Geometry: final body of the model. Coordinates: model frame, mm. Face numbers are marked on the shaded views. A direction names the side the tool comes from. Give positions to 0.01 mm unless a question says otherwise; leave off trailing zeros. Loops run counter-clockwise (first coordinate to the right, second up) from the corner with the lowest first, then second, coordinate; pieces in that order, holes last. Notation, with made-up numbers: (31, 0.5) -> (67, 0.5) arc R28 cw to (67, 18.5) -> close; hole circle Ø9 at (8, 85). An arc over 180 degrees is marked (long way). One line per item, written item: value. Start each with the question number.
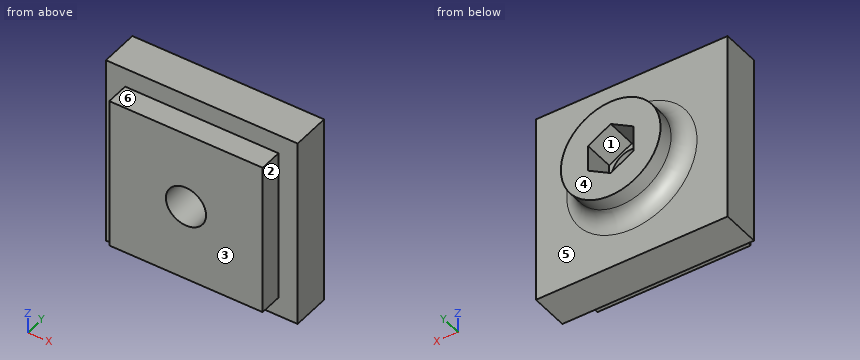
from build123d import *

# Parameters (mm, degrees)
SKETCH2_W               = 25
SKETCH2_H               = 25
BOSS_EXTRUDE1_DEPTH     = 5
SKETCH3_W               = 20
SKETCH3_H               = 20
BOSS_EXTRUDE2_DEPTH     = 3
SKETCH4_R               = 6.5
BOSS_EXTRUDE3_DEPTH     = 4
CUT_EXTRUDE1_DEPTH      = 22.365860619
CUT_EXTRUDE1_DEPTH_BACK = 22.365860619
SKETCH5_R               = 2.62
CUT_EXTRUDE2_DEPTH      = 4
FILLET1_R               = 2


with BuildPart() as part:
    # Sketch2 → Boss-Extrude1 (new body)
    with BuildSketch(Plane(origin=(0, 0, 0), x_dir=(1, 0, 0), z_dir=(0, 1, 0))):
        Rectangle(SKETCH2_W, SKETCH2_H)
    extrude(amount=BOSS_EXTRUDE1_DEPTH)

    # Sketch3 → Boss-Extrude2 (add)
    with BuildSketch(Plane.XZ):
        Rectangle(SKETCH3_W, SKETCH3_H)
    extrude(amount=BOSS_EXTRUDE2_DEPTH)

    # Sketch4 → Boss-Extrude3 (add)
    with BuildSketch(Plane(origin=(0, 5, 0), x_dir=(1, 0, 0), z_dir=(0, 1, 0))):
        with Locations(Location((0, 0, 0), (0, 0, 270))):
            Circle(SKETCH4_R)
    extrude(amount=BOSS_EXTRUDE3_DEPTH)

    # Sketch5 → Cut-Extrude1 (cut, two sides: drawn at the far end of the back side and taken through both)
    with BuildSketch(Plane(origin=(0, 9, 0), x_dir=(1, 0, 0), z_dir=(0, 1, 0)).offset(-CUT_EXTRUDE1_DEPTH_BACK)):
        with Locations(Location((0, 0, 0), (0, 0, 270))):
            Circle(SKETCH5_R)
    extrude(amount=CUT_EXTRUDE1_DEPTH + CUT_EXTRUDE1_DEPTH_BACK, mode=Mode.SUBTRACT)

    # Sketch6 → Cut-Extrude2 (cut)
    with BuildSketch(Plane(origin=(0, 9, 0), x_dir=(1, 0, 0), z_dir=(0, 1, 0))):
        Polygon((0, 3.406366588), (-2.95, 1.703183294), (-2.95, -1.703183294), (0, -3.406366588), (2.95, -1.703183294), (2.95, 1.703183294), align=None)
    extrude(amount=-CUT_EXTRUDE2_DEPTH, mode=Mode.SUBTRACT)

    # Fillet1
    fillet1_edges = [part.edges().sort_by_distance(p)[0] for p in [
        (0, 5, -6.5),
    ]]
    fillet(fillet1_edges, radius=FILLET1_R)


solid = part.part
Item 1: Section D-D, the plane z = -9.25. Output: boundary loops of the cut face in (x, y).
Item 2: Access query for the marked faces 4, 5 and 6. Directions: +Z, -Z, +X, -X, +Y, -Y. A direction counts if a zero-diameter tool reaches every point of the face in a straight line with its end or side. Return the directions, or none.
Item 3: Section A-A, the plane z = 0. Output: boundary loops of the cut face in (x, y).
Item 4: Mould query, pull axis X, two halves, no side actions, for the marked faces 1, 2 and 3. Classes: pulls with the +X half, pulls with the -X half, needs draft (parallel to the pull), parting line crosses it, or undercut.
Item 5: Section C-C, the plane y = 7.75. Output: boundary loops of the cut face in (x, z).
Item 6: Pin query (flat end, axial travel): pin 1 (2.5 mm diameter, centred on x = -2, y = -2, fed in from -Z); pin 2 (3.5 mm diameter, centred on y = 7, z = 0, fed in from -X); pin 3 (1.7 mm diameter, centred on y = 7.5, z = 0, fed in from +X). Return the tip coordinate at first contact, or that it passes through.
Item 7: Ray query, line 1 along Z through (x, y) = (0, 2.5); line 2 along Y through (x, z) = (-6.75, 5.75). Return the intervals inside material, ascending. Write a range as [from, to].
Item 8: Section B-B, the plane x = 9.5. Output: boundary loops of the cut face in (y, z).
Geometry check:
1. outline: (-12.5, 0) -> (-10, 0) -> (-10, -3) -> (10, -3) -> (10, 0) -> (12.5, 0) -> (12.5, 5) -> (-12.5, 5) -> close
2. face 4: +Z, -Z, +X, -X, +Y
2. face 5: +Y
2. face 6: +Z, +X, -X, -Y
3. outline: (-12.5, 0) -> (-10, 0) -> (-10, -3) -> (-2.62, -3) -> (-2.62, 5) -> (-2.95, 5) -> (-2.95, 9) -> (-6.5, 9) -> (-6.5, 7) arc R2 cw to (-8.5, 5) -> (-12.5, 5) -> close; (2.62, -3) -> (10, -3) -> (10, 0) -> (12.5, 0) -> (12.5, 5) -> (8.5, 5) arc R2 cw to (6.5, 7) -> (6.5, 9) -> (2.95, 9) -> (2.95, 5) -> (2.62, 5) -> close
4. face 1: undercut
4. face 2: pulls with the +X half
4. face 3: needs draft
5. outline: circle Ø13 at (0, 0); hole (-2.95, -1.7) -> (0, -3.41) -> (2.95, -1.7) -> (2.95, 1.7) -> (0, 3.41) -> (-2.95, 1.7) -> close
6. pin 1: stops at z = -10
6. pin 2: stops at x = -7.53
6. pin 3: stops at x = 6.53
7. line 1: z = [-12.5, -2.62], [2.62, 12.5]
7. line 2: y = [-3, 5]
8. outline: (-3, -10) -> (0, -10) -> (0, -12.5) -> (5, -12.5) -> (5, 12.5) -> (0, 12.5) -> (0, 10) -> (-3, 10) -> close
